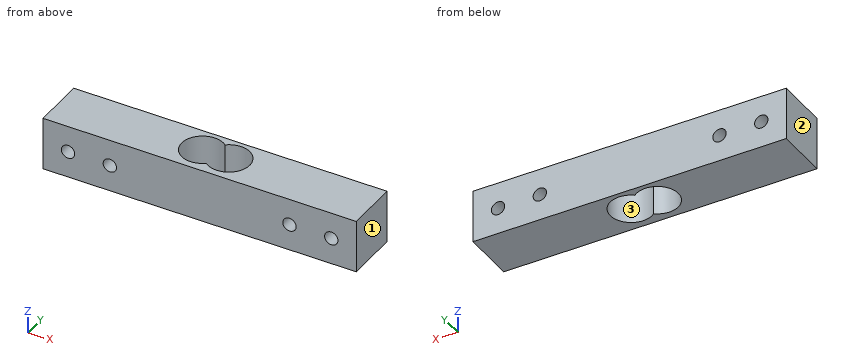
```python
from build123d import *

# Parameters (mm, degrees)
SKETCH2_W           = 75
SKETCH2_H           = 12.7
BOSS_EXTRUDE1_DEPTH = 12.7
CUT_EXTRUDE1_DEPTH  = 12.7
SKETCH4_R           = 1.6
CUT_EXTRUDE2_DEPTH  = 13.7


with BuildPart() as part:
    # Sketch2 → Boss-Extrude1 (new body)
    with BuildSketch(Plane(origin=(0, 0, 0), x_dir=(1, 0, 0), z_dir=(0, 1, 0))):
        with Locations((11.2745, 0.22225)):
            Rectangle(SKETCH2_W, SKETCH2_H)
    extrude(amount=BOSS_EXTRUDE1_DEPTH)

    # Sketch3 → Cut-Extrude1 (cut)
    with BuildSketch(Plane.XY.offset(6.12775)):
        with BuildLine():
            ThreePointArc((11.2745, 10.531229249), (3.1245, 6.648253585), (11.2745, 2.765277922))
            ThreePointArc((11.2745, 2.765277922), (19.4245, 6.648253585), (11.2745, 10.531229249))
        make_face()
    extrude(amount=-CUT_EXTRUDE1_DEPTH, mode=Mode.SUBTRACT)

    # Sketch4 → Cut-Extrude2 (cut, through all)
    with BuildSketch(Plane(origin=(0, 12.7, 0), x_dir=(1, 0, 0), z_dir=(0, 1, 0))):
        with Locations((-20.2255, 0.22225)):
            Circle(SKETCH4_R)
        with Locations((-10.2255, 0.22225)):
            Circle(SKETCH4_R)
        with Locations((32.7745, 0.22225)):
            Circle(SKETCH4_R)
        with Locations((42.7745, 0.22225)):
            Circle(SKETCH4_R)
    extrude(amount=-CUT_EXTRUDE2_DEPTH, mode=Mode.SUBTRACT)


solid = part.part
```
Geometry check sheet. Reference: the model listing, model coordinates, mm. Face numbers are marked on the shaded views. Give positions to 0.01 mm unless a question says otherwise; leave off trailing zeros. Write each loop counter-clockwise with the first axis right and the second up, starting at its lowest first coordinate (ties: lowest second). Pieces come first, ordered by that corner, then holes.
1) Release check for a two-part mould opening along X. For the marked faces 1, 2 and 3 record: pulls with the +X half, pulls with the -X half, needs draft (parallel to the pull), parting line crosses it, or undercut.
2) Section check C-C, the plane z = 3. Record the boundary of the cut face in (x, y), and give its area (3 significant figures).
3) Section check B-B, the plane x = 10. Record the boundary of the cut face in (y, z).
4) Section check D-D, the plane x = 32. Record the boundary of the cut face in (y, z), and give its area (3 significant figures).
5) Section check A-A, the plane y = 5.5. Record the boundary of the cut face in (x, z), and give its area (3 significant figures).
6) Material ranges on L1, parallel to X at y = 9.5, z = 0.5; L2, parallel to X at y = 9.25, z = -1.25; L3, parallel to Y at x = 7, z = -3.25, recorded low to high.
Computed:
1. face 1: pulls with the +X half
1. face 2: pulls with the -X half
1. face 3: undercut
2. outline: (-26.23, 0) - (48.77, 0) - (48.77, 12.7) - (-26.23, 12.7) - close; hole (11.27, 2.77) arc R5 ccw (long way) to (11.27, 10.53) arc R5 ccw (long way) to start
2. area: 815 mm2
3. outline: (0, -6.57) - (2.01, -6.57) - (2.01, 6.13) - (0, 6.13) - close; (11.28, -6.57) - (12.7, -6.57) - (12.7, 6.13) - (11.28, 6.13) - close
4. outline: (0, -6.57) - (12.7, -6.57) - (12.7, -1.62) - (0, -1.62) - close; (0, 1.18) - (12.7, 1.18) - (12.7, 6.13) - (0, 6.13) - close
4. area: 126 mm2
5. outline: (-26.23, -6.57) - (3.26, -6.57) - (3.26, 6.13) - (-26.23, 6.13) - close; (19.29, -6.57) - (48.77, -6.57) - (48.77, 6.13) - (19.29, 6.13) - close; hole circle Ø3.2 at (-20.23, -0.22); hole circle Ø3.2 at (-10.23, -0.22); hole circle Ø3.2 at (32.77, -0.22); hole circle Ø3.2 at (42.77, -0.22)
5. area: 717 mm2
6. L1: x = -26.23 to -21.65, -18.8 to -11.65, -8.8 to 4.02, 18.53 to 31.35, 34.2 to 41.35, 44.2 to 48.77
6. L2: x = -26.23 to -21.45, -19 to -11.45, -9 to 3.85, 18.69 to 31.55, 34 to 41.55, 44 to 48.77
6. L3: y = 0 to 1.78, 11.52 to 12.7
